Geometry check sheet. Reference: drawing and pictorial views, mm from the part's lowest x, y, z. Coordinates: 2 decimals unless noted, no trailing zeros. Write each loop counter-clockwise with the first axis right and the second up, starting at its lowest first coordinate (ties: lowest second). Pieces come first, ordered by that corner, then holes. Notation, with made-up numbers: (43, 36.25) -> (77, 36.25) arc R22 cw to (77, 43.25) -> close; hole circle Ø5 at (43.25, 82). An arc over 180 degrees is marked (long way). Use a Markdown table: item, result. Add a question column.
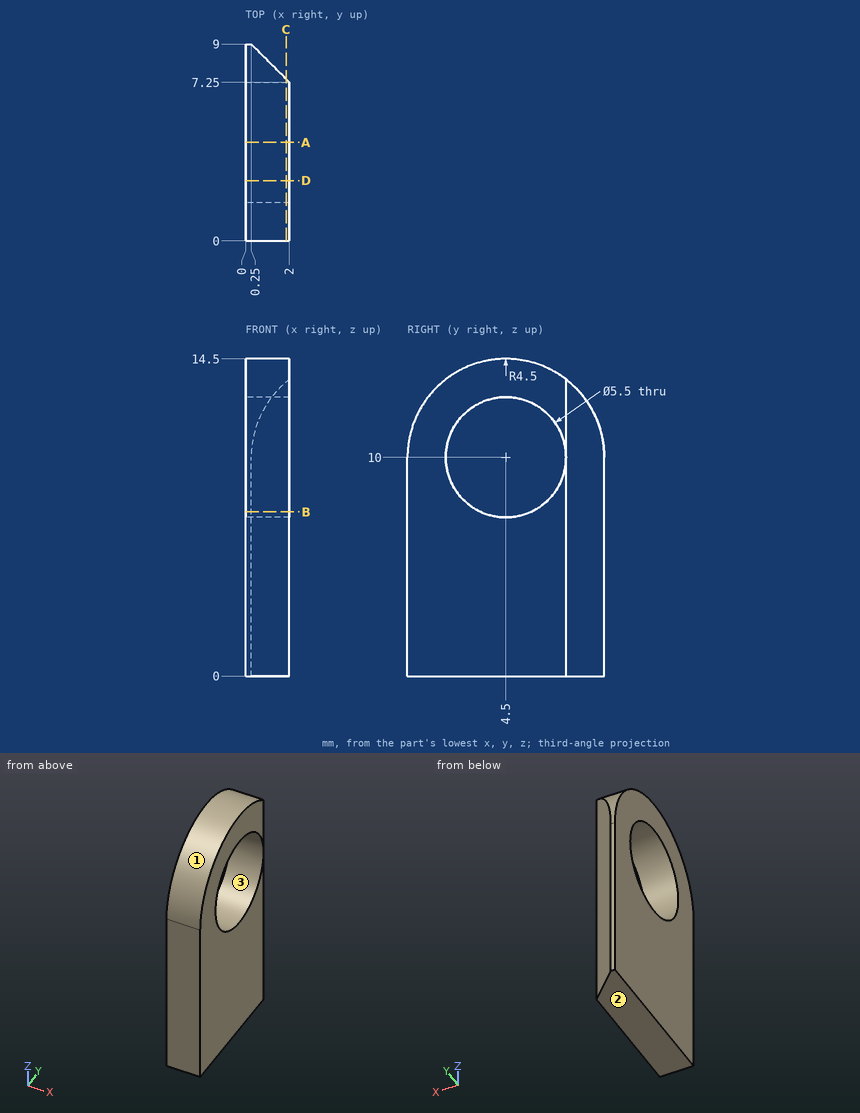
1) Cross-section at A-A on y = 4.5. Record the boundary of the cut face in (x, z), then the cut area to 3 significant figures.
2) Thickness scan on L1, parallel to Z at x = 1.3, y = 4.5; L2, parallel to Z at x = 1.4, y = 2.25; L3, parallel to Y at x = 1.45, z = 11.25. Record the ranges inside material, lowest first.
3) Cross-section at B-B on z = 7.5. Record the boundary of the cut face in (x, y).
4) Cross-section at C-C on x = 1.85. Record the boundary of the cut face in (y, z).
5) Release check for a two-part mould opening along Z. For the marked faces 1, 2 and 3 record: released by +Z, released by -Z, zero draft, split by the parting line, or undercut.
6) Gauge pin test, flat end, axial feed: pin 1 (4.5 mm diameter, centred on y = 4.5, z = 10, fed in from -X). Record the tip position at first contact, or that the pin passes through.
7) Cross-section at D-D on y = 2.75. Record the boundary of the cut face in (x, z), then the cut area to 3 significant figures.
Returned:
| question | item | result |
|---|---|---|
| 1 | outline | (0, 0) -> (2, 0) -> (2, 7.25) -> (0, 7.25) -> close; (0, 12.75) -> (2, 12.75) -> (2, 14.5) -> (0, 14.5) -> close |
| 1 | area | 18.0 mm² |
| 2 | L1 | z = 0 to 7.25, 12.75 to 14.5 |
| 2 | L2 | z = 0 to 8.42, 11.58 to 13.9 |
| 2 | L3 | y = 0.18 to 2.05, 6.95 to 7.8 |
| 3 | outline | (0, 0) -> (2, 0) -> (2, 3.35) -> (0, 3.35) -> close; (0, 5.65) -> (2, 5.65) -> (2, 7.25) -> (0.25, 9) -> (0, 9) -> close |
| 4 | outline | (0, 0) -> (7.4, 0) -> (7.4, 13.44) arc R4.5 ccw to (0, 10) -> close; hole circle Ø5.5 at (4.5, 10) |
| 5 | face 1 | released by +Z |
| 5 | face 2 | released by -Z |
| 5 | face 3 | undercut |
| 6 | pin 1 | passes through |
| 7 | outline | (0, 0) -> (2, 0) -> (2, 7.88) -> (0, 7.88) -> close; (0, 12.12) -> (2, 12.12) -> (2, 14.15) -> (0, 14.15) -> close |
| 7 | area | 19.8 mm² |
